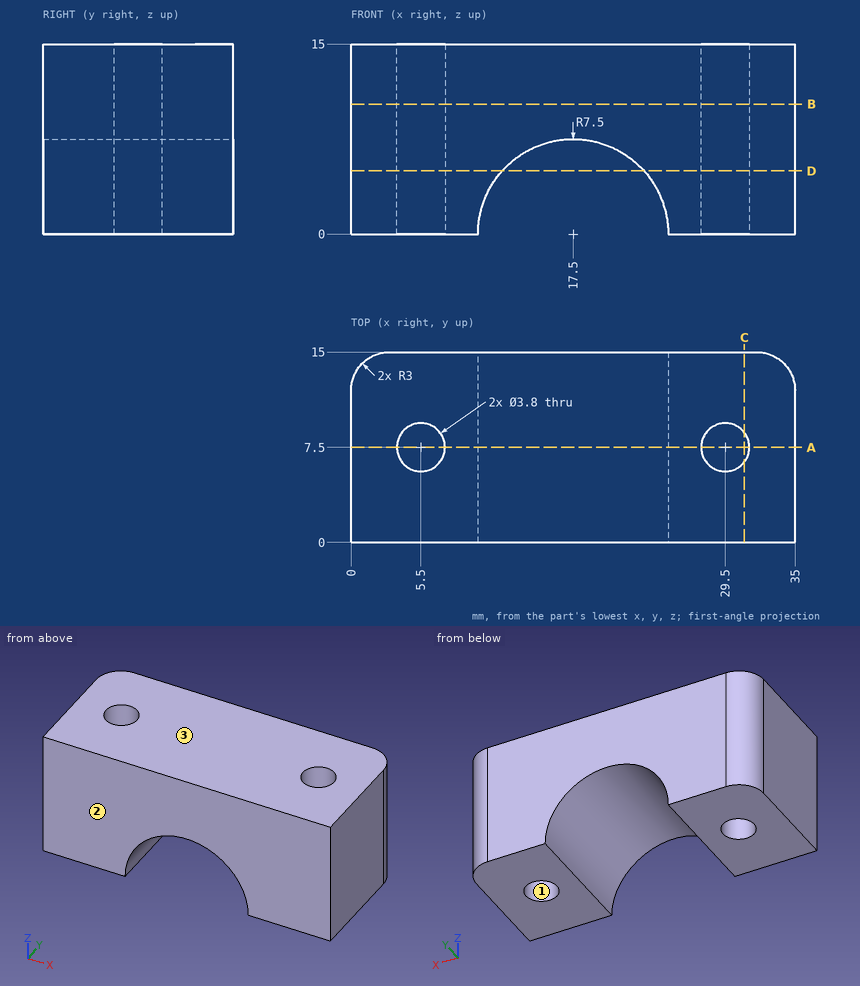
Geometry check sheet. Reference: drawing and pictorial views, mm from the part's lowest x, y, z. Give positions to 0.01 mm unless a question says otherwise; leave off trailing zeros. Loops run counter-clockwise (first coordinate to the right, second up) from the corner with the lowest first, then second, coordinate; pieces in that order, holes last. Notation, with made-up numbers: (82.5, 41.5) - (97.5, 41.5) arc R24 cw to (97.5, 68.5) - close; hole circle Ø8 at (81, 33.25). An arc over 180 degrees is marked (long way). Use CSV: the item, a comma, the result in double quotes. Start each with the question number.
Q1. Section check B-B, the plane z = 10.25. Record the cut outline in (x, y), and give its area (3 significant figures).
Q2. Release check for a two-part mould opening along Y. For the marked faces 1, 2 and 3 record: +Y half, -Y half, draft (parallel to the pull), parting line (faces both ways), or undercut.
Q3. Go/stop test with a flat-tipped pin: pin 1 Ø4.5 at (x, y) = (5.5, 7.5) entering from -Z. Record where the tip stops, or that it passes through.
Q4. Section check D-D, the plane z = 5. Record the cut outline in (x, y), and give its area (3 significant figures).
Q5. Scan lines: probe 1 along Y at (x, z) = (29.5, 6.25); probe 2 along X at (y, z) = (8.5, 13); probe 3 along X at (y, z) = (11.5, 3.25). Record each from-to range of solid material in increasing order. Write a range as from..to.
Q6. Section check A-A, the plane y = 7.5. Record the cut outline in (x, z).
Q7. Section check C-C, the plane x = 31. Record the cut outline in (y, z).
Findings below:
1,outline,"(0, 0) - (35, 0) - (35, 12) arc R3 ccw to (32, 15) - (3, 15) arc R3 ccw to (0, 12) - close; hole circle Ø3.8 at (5.5, 7.5); hole circle Ø3.8 at (29.5, 7.5)"
1,area,"498 mm^2"
2,face 1,"undercut"
2,face 2,"-Y half"
2,face 3,"draft"
3,pin 1,"stops at z = 0"
4,outline,"(0, 0) - (11.91, 0) - (11.91, 15) - (3, 15) arc R3 ccw to (0, 12) - close; (23.09, 0) - (35, 0) - (35, 12) arc R3 ccw to (32, 15) - (23.09, 15) - close; hole circle Ø3.8 at (5.5, 7.5); hole circle Ø3.8 at (29.5, 7.5)"
4,area,"331 mm^2"
5,probe 1,"y = 0..5.6, 9.4..15"
5,probe 2,"x = 0..3.88, 7.12..27.88, 31.12..35"
5,probe 3,"x = 0..10.74, 24.26..35"
6,outline,"(0, 0) - (3.6, 0) - (3.6, 15) - (0, 15) - close; (7.4, 0) - (10, 0) arc R7.5 cw to (25, 0) - (27.6, 0) - (27.6, 15) - (7.4, 15) - close; (31.4, 0) - (35, 0) - (35, 15) - (31.4, 15) - close"
7,outline,"(0, 0) - (6.33, 0) - (6.33, 15) - (0, 15) - close; (8.67, 0) - (15, 0) - (15, 15) - (8.67, 15) - close"
